Check sheet for the drawn part. Datum: minimum x, y, z corner. Units: mm. A direction names the side the tool comes from. Coordinates: 2 decimals unless noted, no trailing zeros. Order: outer loops, then holes, each group sorted by start corner. A loop starts at its lowest first (then second) coordinate and runs counter-clockwise, first axis right, second up.
1. Cross-section at C-C (z = 8.5). Enter the section's corners in (x, y).
2. Draft check along Y on the marked faces 1, 2 and 3. Enter one of: released by +Y, released by -Y, zero draft, split by the parting line, or undercut.
3. Cross-section at D-D (z = 29.5). Enter the section's corners in (x, y), then the cut area to 3 significant figures.
4. Cross-section at B-B (x = 40). Enter the section's corners in (y, z), then the cut area to 3 significant figures.
5. Gauge pin test, flat ends, axial feed: pin 1 Ø1.5 at (x, z) = (17.5, 24) entering from -Y; pin 2 Ø1.5 at (x, z) = (47, 25.5) entering from -Y; pin 3 Ø8 at (x, z) = (49, 29) entering from -Y. Record the tip position at first contact, or that the pin passes through.
6. Set-up check for the marked faces 4 and 5: record each of +Z, -Z, +X, -X, +Y, -Y from which the full face is reachable in a straight line by a thin tool's end or side.
7. Cross-section at A-A (y = 35). Enter the section's corners in (x, z), then the cut area to 3 significant figures.
8. Thickness scan on line 1 (Y direction, x = 40, z = 30); line 2 (X direction, y = 31, z = 2) (1 decimal); line 3 (Y direction, x = 50.5, z = 23). Record the ranges inside material, lowest first.
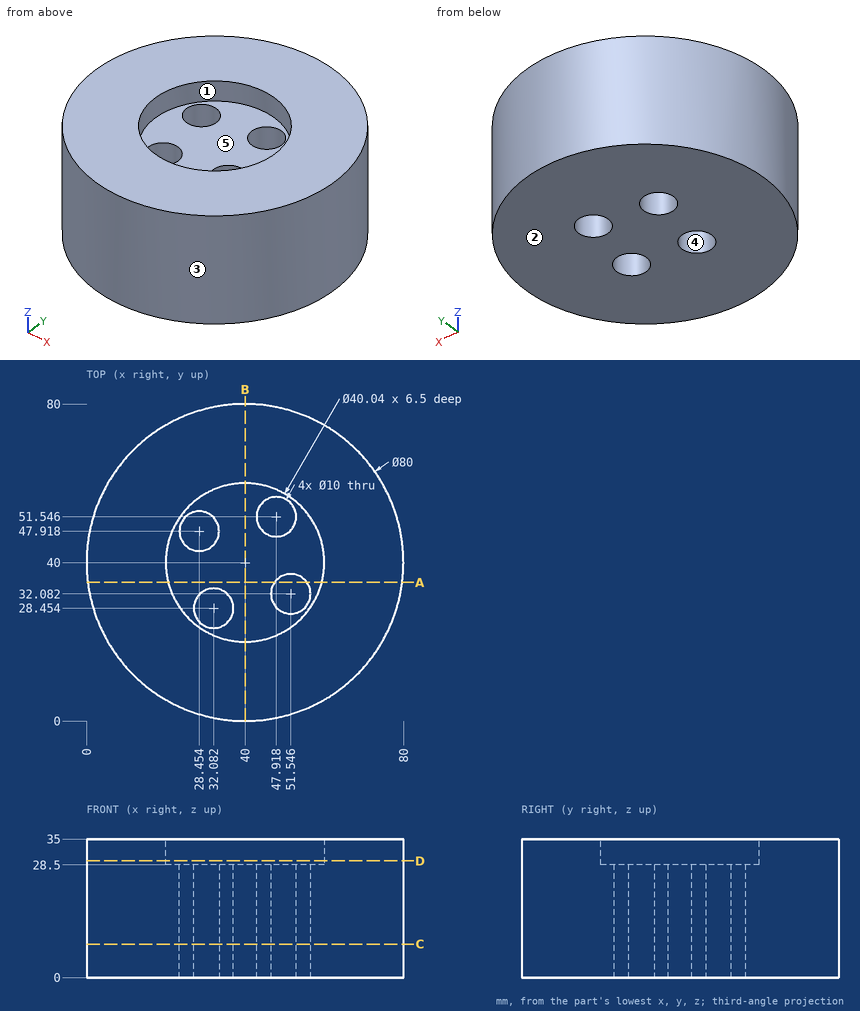
Data:
1. outline: circle Ø80 at (40, 40); hole circle Ø10 at (28.45, 47.92); hole circle Ø10 at (32.08, 28.45); hole circle Ø10 at (47.92, 51.55); hole circle Ø10 at (51.55, 32.08)
2. face 1: undercut
2. face 2: zero draft
2. face 3: split by the parting line
3. outline: circle Ø80 at (40, 40); hole circle Ø40.04 at (40, 40)
3. area: 3,770 mm2
4. outline: (0, 0) - (80, 0) - (80, 35) - (60.02, 35) - (60.02, 28.5) - (19.98, 28.5) - (19.98, 35) - (0, 35) - close
4. area: 2,540 mm2
5. pin 1: stops at y = 6.43
5. pin 2: stops at y = 0.49
5. pin 3: stops at y = 0.31
6. face 4: +Z, -Z
6. face 5: +Z
7. outline: (0.31, 0) - (47.49, 0) - (47.49, 28.5) - (20.61, 28.5) - (20.61, 35) - (0.31, 35) - close; (55.61, 0) - (79.69, 0) - (79.69, 35) - (59.39, 35) - (59.39, 28.5) - (55.61, 28.5) - close
7. area: 2,290 mm2
8. line 1: y = 0 to 19.98, 60.02 to 80
8. line 2: x = 1 to 27.8, 36.4 to 46.7, 56.4 to 79
8. line 3: y = 1.4 to 27.19, 36.97 to 47.26, 55.83 to 78.6
